Verification items for this drawing (mm, ordinates from the low corner). Give positions to 0.01 mm unless a question says otherwise; leave off trailing zeros. Write each loop counter-clockwise with the first axis right and the second up, starting at its lowest first coordinate (ties: lowest second). Pieces come first, ordered by that corner, then holes. Notation, with made-up numbers: (-25.75, -18) -> (-0.75, -18) arc R8 ccw to (-0.75, -7) -> close; hole circle Ø2 at (-29.75, 87). An arc over 180 degrees is marked (long way). Use one line per item in the form item = value. Start each with the question number.
(1) Section check B-B, the plane z = 25. Record the cut outline in (x, y) (1 decimal).
(2) Depth check by flat-ended pin: pin 1 Ø10 at (x, y) = (8.5, 4) entering from +Z; pin 2 Ø10 at (x, z) = (16.5, 7.5) entering from -Y (1 decimal); pin 3 Ø6 at (x, z) = (13.5, 15) entering from -Y. Enter the tip coordinate at first touch or a pass-through.
(3) Release check for a two-part mould opening along X. For the marked faces 1, 2, 3 and 4 record: pulls with the +X half, pulls with the -X half, needs draft (parallel to the pull), parting line crosses it, or undercut.
(4) Section check C-C, the plane x = 1.5. Record the cut outline in (y, z).
(5) Section check D-D, the plane z = 21. Record the cut outline in (x, y) (1 decimal).
(6) Scan lines: L1, parallel to X at y = 2.5, z = 21.5; L2, parallel to Y at x = 17.5, z = 18; L3, parallel to Z at x = 1.25, y = 13.5 (1 decimal). Record each from-to range of solid material in increasing order.
(7) Section check A-A, the plane y = 1. Record the cut outline in (x, z).
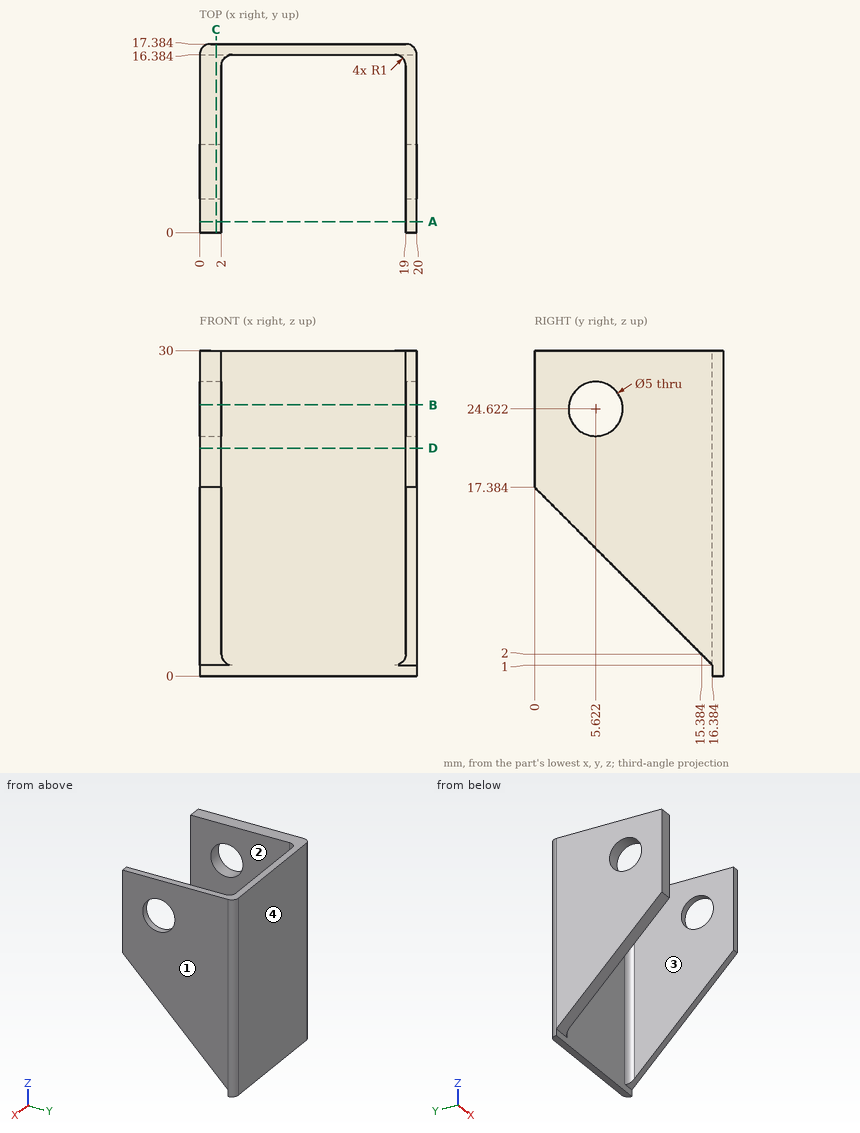
Completed:
q1.outline = (0, 0) -> (2, 0) -> (2, 3.2) -> (0, 3.2) -> close; (0, 8.1) -> (2, 8.1) -> (2, 15.4) arc R1 cw to (3, 16.4) -> (18, 16.4) arc R1 cw to (19, 15.4) -> (19, 8.1) -> (20, 8.1) -> (20, 16.4) arc R1 ccw to (19, 17.4) -> (1, 17.4) arc R1 ccw to (0, 16.4) -> close; (19, 0) -> (20, 0) -> (20, 3.2) -> (19, 3.2) -> close
q2.pin_1 = through
q2.pin_2 = 5.6
q2.pin_3 = 16.38
q3.face_1 = pulls with the +X half
q3.face_2 = undercut
q3.face_3 = undercut
q3.face_4 = needs draft
q4.outline = (0, 17.38) -> (16.38, 1) -> (16.38, 0) -> (17.38, 0) -> (17.38, 30) -> (0, 30) -> close; hole circle Ø5 at (5.62, 24.62)
q5.outline = (0, 0) -> (2, 0) -> (2, 15.4) arc R1 cw to (3, 16.4) -> (18, 16.4) arc R1 cw to (19, 15.4) -> (19, 0) -> (20, 0) -> (20, 16.4) arc R1 ccw to (19, 17.4) -> (1, 17.4) arc R1 ccw to (0, 16.4) -> close
q6.L1 = 0 to 2, 19 to 20
q6.L2 = 16.38 to 17.38
q6.L3 = 3.9 to 30
q7.outline = (0, 16.38) -> (2, 16.38) -> (2, 30) -> (0, 30) -> close; (19, 16.38) -> (20, 16.38) -> (20, 30) -> (19, 30) -> close
